from build123d import *

# Parameters (mm, degrees)
SKETCH1_W           = 30
SKETCH1_H           = 31
BOSS_EXTRUDE1_DEPTH = 10
SKETCH2_W           = 4
SKETCH2_H           = 10
CUT_EXTRUDE1_DEPTH  = 10
CHAMFER1_SIZE       = 4
SKETCH3_R           = 2.25
CUT_EXTRUDE2_DEPTH  = 15
CHAMFER2_SIZE       = 1
SKETCH4_R           = 10
CUT_EXTRUDE3_DEPTH  = 24.774986856
BOSS_EXTRUDE2_DEPTH = 19
CHAMFER3_SIZE       = 4
SKETCH6_W           = 28
SKETCH6_H           = 10
CUT_EXTRUDE4_DEPTH  = 15
FILLET1_R           = 5
SKETCH7_R           = 1.75
CUT_EXTRUDE5_DEPTH  = 68.825142831
FILLET2_R           = 2
SKETCH8_R           = 2
CUT_EXTRUDE6_DEPTH  = 60.306407782
SKETCH9_R           = 7.5
CUT_EXTRUDE7_DEPTH  = 5
BOSS_EXTRUDE3_DEPTH = 5
CHAMFER4_SIZE       = 3


with BuildPart() as part:
    # Sketch1 → Boss-Extrude1 (new body)
    with BuildSketch(Plane.XY):
        Rectangle(SKETCH1_W, SKETCH1_H)
    extrude(amount=BOSS_EXTRUDE1_DEPTH)

    # Sketch2 → Cut-Extrude1 (cut)
    with BuildSketch(Plane.XZ.offset(15.5)):
        with Locations((-13, 5)):
            Rectangle(SKETCH2_W, SKETCH2_H)
        with Locations((13, 5)):
            Rectangle(SKETCH2_W, SKETCH2_H)
    extrude(amount=-CUT_EXTRUDE1_DEPTH, mode=Mode.SUBTRACT)

    # Chamfer1
    chamfer1_edges = [part.edges().sort_by_distance(p)[0] for p in [
        (11, -5.5, 5),
        (-11, -5.5, 5),
    ]]
    chamfer(chamfer1_edges, length=CHAMFER1_SIZE - 0.0001)  # a hair under: the kernel refuses the full size

    # Sketch3 → Cut-Extrude2 (cut)
    with BuildSketch(Plane.XZ.offset(15.5)):
        with Locations(Location((-7.5, 3.5, 0), (0, 0, 270))):
            Circle(SKETCH3_R)
        with Locations(Location((0, 3.5, 0), (0, 0, 270))):
            Circle(SKETCH3_R)
        with Locations(Location((7.5, 3.5, 0), (0, 0, 270))):
            Circle(SKETCH3_R)
    extrude(amount=-CUT_EXTRUDE2_DEPTH, mode=Mode.SUBTRACT)

    # Chamfer2
    chamfer2_edges = [part.edges().sort_by_distance(p)[0] for p in [
        (-7.5, -15.5, 5.75),
        (0, -15.5, 5.75),
        (7.5, -15.5, 5.75),
    ]]
    chamfer(chamfer2_edges, length=CHAMFER2_SIZE)

    # Sketch4 → Cut-Extrude3 (cut, through all)
    with BuildSketch(Plane(origin=(0, 0, 0), x_dir=(-1, 0, 0), z_dir=(0, 0, -1))):
        with Locations((0, 4.5)):
            Circle(SKETCH4_R)
    extrude(amount=-CUT_EXTRUDE3_DEPTH, mode=Mode.SUBTRACT)

    # Sketch5 → Boss-Extrude2 (add, symmetric)
    with BuildSketch(Plane(origin=(0, 0, 0), x_dir=(0, 0, -1), z_dir=(1, 0, 0))):
        Polygon((-10, 14.5), (-20, 24.5), (-20, 52.5), (-10, 52.5), (-10, 25.5), (0, 15.5), align=None)
    extrude(amount=BOSS_EXTRUDE2_DEPTH, both=True)

    # Chamfer3
    chamfer3_edges = [part.edges().sort_by_distance(p)[0] for p in [
        (-19, 15, 5),
        (19, 15, 5),
    ]]
    chamfer(chamfer3_edges, length=CHAMFER3_SIZE - 0.0001)  # a hair under: the kernel refuses the full size

    # Sketch6 → Cut-Extrude4 (cut)
    with BuildSketch(Plane(origin=(0, 52.5, 0), x_dir=(1, 0, 0), z_dir=(0, 1, 0))):
        with Locations((0, -15)):
            Rectangle(SKETCH6_W, SKETCH6_H)
    extrude(amount=-CUT_EXTRUDE4_DEPTH, mode=Mode.SUBTRACT)

    # Fillet1
    fillet1_edges = [part.edges().sort_by_distance(p)[0] for p in [
        (16.5, 52.5, 10),
        (16.5, 52.5, 20),
        (-16.5, 52.5, 10),
        (-16.5, 52.5, 20),
    ]]
    fillet(fillet1_edges, radius=FILLET1_R - 0.0001)  # a hair under: the kernel refuses the full size

    # Sketch7 → Cut-Extrude5 (cut, through all)
    with BuildSketch(Plane(origin=(19, 0, 0), x_dir=(0, 0, -1), z_dir=(1, 0, 0))):
        with Locations((-15, 47.5)):
            Circle(SKETCH7_R)
    extrude(amount=-CUT_EXTRUDE5_DEPTH, mode=Mode.SUBTRACT)

    # Fillet2
    fillet2_edges = [part.edges().sort_by_distance(p)[0] for p in [
        (19, 36.00005, 20),
        (19, 51.035563195, 18.535563195),
        (19, 51.035563195, 11.464436805),
        (-19, 36.00005, 20),
        (-19, 51.035563195, 18.535563195),
        (-19, 51.035563195, 11.464436805),
        (-19, 36.50005, 10),
        (19, 36.50005, 10),
    ]]
    fillet(fillet2_edges, radius=FILLET2_R)

    # Sketch8 → Cut-Extrude6 (cut, through all)
    with BuildSketch(Plane.XY.offset(20)):
        with Locations((0, 32.5)):
            Circle(SKETCH8_R)
    extrude(amount=-CUT_EXTRUDE6_DEPTH, mode=Mode.SUBTRACT)

    # Sketch9 → Cut-Extrude7 (cut)
    with BuildSketch(Plane.XY.offset(20)):
        with Locations((0, 32.5)):
            Circle(SKETCH9_R)
    extrude(amount=-CUT_EXTRUDE7_DEPTH, mode=Mode.SUBTRACT)

    # Sketch10 → Boss-Extrude3 (add)
    with BuildSketch(Plane(origin=(15, 0, 0), x_dir=(0, 0, -1), z_dir=(1, 0, 0))):
        Polygon((-10, -5.5), (-18, 22.5), (-10, 14.5), align=None)
    boss_extrude3 = extrude(amount=-BOSS_EXTRUDE3_DEPTH)

    # Mirror1: Boss-Extrude3 across plane
    add(boss_extrude3.mirror(Plane(origin=(0, 0, 0), x_dir=(0, 0, 1), z_dir=(1, 0, 0))))

    # Chamfer4
    chamfer4_edges = [part.edges().sort_by_distance(p)[0] for p in [
        (0, -15.5, 10),
    ]]
    chamfer(chamfer4_edges, length=CHAMFER4_SIZE)


solid = part.part
Geometry check sheet. Reference: the model listing, model coordinates, mm. A direction names the side the tool comes from. Round coordinates to 2 decimals unless told otherwise and drop trailing zeros. Order: outer loops, then holes, each group sorted by start corner. A loop starts at its lowest first (then second) coordinate and runs counter-clockwise, first axis right, second up. Notation, with made-up numbers: M -16.75,-6.75 L 34.25,-6.75 A20 ccw 34.25,27.25 Z; hole C 38.5,86 d2. An arc over 180 degrees is marked long. Answer in a Markdown table with one row per item. Add a question column.
Item 1: Sectioned sample at A-A, the plane y = 32.5. Enter the section's corners in (x, z).
Item 2: Sectioned sample at D-D, the plane y = 10.5. Enter the section's corners in (x, z), plus the area to 3 significant figures.
Item 3: Sectioned sample at B-B, the plane y = -7.5. Enter the section's corners in (x, z), plus the area to 3 significant figures.
Item 4: Depth check by flat-ended pin: pin 1 Ø3 at (x, y) = (0, 32.5) entering from -Z; pin 2 Ø11 at (x, z) = (-6, 14) entering from +Y; pin 3 Ø2.5 at (x, z) = (0, 3.5) entering from -Y; pin 4 Ø1 at (x, y) = (5.5, 35.5) entering from +Z. Enter the tip coordinate at first touch or a pass-through.
Item 5: Material ranges on L1, parallel to X at y = 32.5, z = 18.25; L2, parallel to X at y = 44.5, z = 13.25; L3, parallel to X at y = -5.5, z = 3.5, recorded low to high. Write a range as [from, to].
Item 6: Draft check along Z on faces 6 (the face through (12.535, 8.304, 13.944)), 7 (the face through (0, 37, 10)), 8 (the face through (0.676, -9.937, 1.354)), 9 (the face through (9.73, -7.6, 3.79)). Enter one of: released by +Z, released by -Z, zero draft, split by the parting line, or undercut.
Item 7: Sectioned sample at C-C, the plane z = 16. State how many separate pieces and enclosed holes the cut face has, plus the area to 3 significant figures.
Item 8: Set-up check for faces 1 (the face through (0, -8, 10)), 2 (the face through (-16.47, 45.79, 15.38)), 3 (the face through (-18.43, 36.35, 10.6)), 4 (the face through (-11, -13, 5)), 5 (the face through (14, 45, 15)): record each of +Z, -Z, +X, -X, +Y, -Y from which the full face is reachable in a straight line by a thin tool's end or side.
Filled in:
| question | item | result |
|---|---|---|
| 1 | outline | M -19,12 A2 ccw -17,10 L -2,10 L -2,15 L -7.5,15 L -7.5,20 L -17,20 A2 ccw -19,18 Z; M 2,10 L 17,10 A2 ccw 19,12 L 19,18 A2 ccw 17,20 L 7.5,20 L 7.5,15 L 2,15 Z |
| 2 | outline | M -15,0 L -8,0 L -8,10 L -10,10 L -10,14.57 L -15,14.57 Z; M 8,0 L 15,0 L 15,14.57 L 10,14.57 L 10,10 L 8,10 Z |
| 2 | area | 186 mm² |
| 3 | outline | M -13,0 L 13,0 L 13,10 L -13,10 Z; hole C -7.5,3.5 d4.5; hole C 0,3.5 d4.5; hole C 7.5,3.5 d4.5 |
| 3 | area | 212 mm² |
| 4 | pin 1 | passes through |
| 4 | pin 2 | stops at y = 37.5 |
| 4 | pin 3 | stops at y = 14.42 |
| 4 | pin 4 | stops at z = 15 |
| 5 | L1 | x = [-18.98, -7.5], [7.5, 18.98] |
| 5 | L2 | x = [-19, -14], [14, 19] |
| 5 | L3 | x = [-15, -9.75], [-5.25, -2.25], [2.25, 5.25], [9.75, 15] |
| 6 | face 6 | released by +Z |
| 6 | face 7 | released by -Z |
| 6 | face 8 | undercut |
| 6 | face 9 | undercut |
| 7 | separate pieces | 3 |
| 7 | enclosed holes | 0 |
| 7 | area | 657 mm² |
| 8 | face 1 | +Z, -Y |
| 8 | face 2 | +X, -X |
| 8 | face 3 | -Z, -X, +Y |
| 8 | face 4 | +Z, -Z, -X, -Y |
| 8 | face 5 | +Z, -Z, +Y |
